For this review, take the finished solid that the model builds, in its own axes (mm). Face numbers are marked on the shaded views. A direction names the side the tool comes from. Round coordinates to 2 decimals unless told otherwise and drop trailing zeros. Write each loop counter-clockwise with the first axis right and the second up, starting at its lowest first coordinate (ties: lowest second). Pieces come first, ordered by that corner, then holes. Notation, with made-up numbers: (-25, 13.25) -> (0, 13.25) arc R12 cw to (0, 36.25) -> close; hole circle Ø10 at (8, 16.5). An arc over 180 degrees is marked (long way). Answer as CSV lines item,"result". Start each with the question number.
Item 1: Take a section at D-D on x = 31. Give the boundary of the cut face in (y, z), then the cut area to 3 significant figures.
Item 2: Take a section at B-B on z = -20. Count the separate pieces of the cut face and the enclosed holes in it, then the cut area to 3 significant figures.
Item 3: Wall thickness on probe 1 along X at (y, z) = (26.8, -20); probe 2 along Z at (x, y) = (21, 30.5); probe 3 along X at (y, z) = (27.5, -30): over which ranges is each line inside the solid? List them lowest first. Write a range as from..to.
Item 4: Mouldability with a two-part tool opening along Z and no side actions: class the marked faces 1, 2, 3 and 4 as +Z half, -Z half, draft (parallel to the pull), parting line (faces both ways), or undercut.
Item 5: For pin 1 Ø5.5 at (x, z) = (112.5, -22) entering from +Y; pin 2 Ø5 at (x, z) = (30.5, -30) entering from +Y; pin 3 Ø2.5 at (x, z) = (111.5, -19.5) entering from -Y; pin 4 Ø20 at (y, z) = (11.5, -22.5) entering from +X, all flat-tipped, find the tip position at first contact; note any pin that passes through.
Item 6: Machinability: for the marked faces 5 and 6, which of the approach directions +Z, -Z, +X, -X, +Y, -Y give a long, thin tool a straight path to every point of the face, cutting with its end or side? Answer none if there is none.
Item 7: Take a section at A-A on y = 2.5. Give the boundary of the cut face in (x, z), then the cut area to 3 significant figures.
Item 8: Take a section at C-C on z = -36.5. Give the boundary of the cut face in (x, y).
Autodesk Inventor part; units mm, degrees
ref_plane "YZ Plane" through (0, 0, 0) normal (1, 0, 0) x (0, 1, 0)
ref_plane "XZ Plane" through (0, 0, 0) normal (0, 1, 0) x (-1, 0, 0)
ref_plane "XY Plane" through (0, 0, 0) normal (0, 0, 1) x (1, 0, 0)
sketch "Sketch1" plane through (0, 0, 0) normal (0, 1, 0) x (-1, 0, 0)
  line L0 (0, 0) -> (-100, 0)
  line L1 (-100, 0) -> (-100, -40)
  line L2 (-100, -40) -> (0, -40)
  line L3 (0, -40) -> (0, 0)
  line L4 (2, -42) -> (-102, -42)
  line L5 (-102, -42) -> (-102, 2)
  line L6 (-102, 2) -> (2, 2)
  line L7 (2, 2) -> (2, -42)
  dimension "Length" = 100
  dimension "Width" = 40
  dimension "Thickness" = 2
extrude "Extrusion1" add sketch "Sketch1" along normal blind 40
sketch "Sketch2" plane through (0, 0, 0) normal (0, -1, 0) x (1, 0, 0)
  line L0 (102, -42) -> (102, 2)
  line L1 (102, 2) -> (-2, 2)
  line L2 (-2, -42) -> (102, -42)
  line L3 (-2, 2) -> (-2, -42)
  point P0 (0, 0)
extrude "Extrusion2" add sketch "Sketch2" along normal blind 2
sketch "Sketch3" plane through (-2, 40, -42) normal (-1, 0, 0) x (0, 0, 1)
  line L0 (0, 0) -> (44, 0)
  line L1 (19.5, -4) -> (24.5, -4)
  line L2 (24.5, -4) -> (24.5, -2)
  line L3 (24.5, -2) -> (19.5, -2)
  line L4 (19.5, -2) -> (19.5, -4)
  line L5 (19.5, -4) -> (24.5, -2) construction
  line L6 (24.5, -4) -> (19.5, -2) construction
  line L7 (22, -3) -> (22, 0) construction
  point P0 (42, -40)
  dimension "d7" = 5
  dimension "d8" = 2
  dimension "d9" = 2
extrude "Extrusion3" cut sketch "Sketch3" against normal up to next
sketch "Sketch4" plane through (102, 40, 2) normal (1, 0, 0) x (0, 0, -1)
  line L0 (14.5, -12) -> (29.5, -12)
  line L1 (29.5, -12) -> (29.5, -10)
  line L2 (29.5, -10) -> (14.5, -10)
  line L3 (14.5, -10) -> (14.5, -12)
  line L4 (14.5, -12) -> (29.5, -10) construction
  line L5 (29.5, -12) -> (14.5, -10) construction
  line L6 (0, 0) -> (44, 0)
  line L7 (22, -11) -> (22, 0) construction
  line L8 (44, 0) -> (0, 0)
  point P0 (2, -40)
  dimension "d12" = 10
  dimension "d13" = 15
  dimension "d14" = 2
extrude "Extrusion4" add sketch "Sketch4" along normal blind 10
sketch "Sketch5" plane through (102, 30, -12.5) normal (0, 1, 0) x (1, 0, 0)
  line L0 (0, 0) -> (0, 15)
  line L1 (0, 0) -> (10, 0)
  line L2 (10, 15) -> (10, 0)
  line L3 (0, 15) -> (10, 15)
  line L4 (10, 0) -> (10, 15)
  arc A0 (10, 0) -> (10, 15) centre (10, 7.5) ccw
  point P0 (-102, -12.5)
extrude "Extrusion5" add sketch "Sketch5" against normal blind 10
sketch "Sketch6" plane through (102, 30, -12.5) normal (0, 1, 0) x (1, 0, 0)
  arc A0 (10, 0) -> (10, 15) centre (10, 7.5) ccw
  point P0 (-102, -12.5)
hole "Hole1" at (112, 30, -20) direction (0, -1, 0) diameter 5.5 end through all
fillet "Fillet1" radius 2 11 edges at (119.5, 30, -20) (107, 30, -12.5) (107, 30, -27.5) (112, 30, -22.75) (119.5, 20, -20) (107, 20, -12.5) (107, 20, -27.5) (102, 25, -27.5) (102, 20, -20) (102, 25, -12.5) (102, 30, -20)
sketch "Sketch7" plane through (102, 20, -12.5) normal (0, -1, 0) x (1, 0, 0)
  circle A0 centre (10, -7.5) radius 2.75
  circle A1 centre (10, -7.5) radius 4 construction
  line L0 (14, -9.8094) -> (10, -12.1188)
  line L1 (10, -12.1188) -> (6, -9.8094)
  line L2 (6, -9.8094) -> (6, -5.1906)
  line L3 (6, -5.1906) -> (10, -2.8812)
  line L4 (10, -2.8812) -> (14, -5.1906)
  line L5 (14, -5.1906) -> (14, -9.8094)
  point P0 (-102, 12.5)
  point P1 (14, -7.5)
  dimension "d27" = 8
extrude "Extrusion6" cut sketch "Sketch7" against normal blind 3.5
equation "\"d5\" = Thickness"
equation "\"d10\" = Thickness"
equation "\"d14\" = Thickness"
properties part number "Casing_Part1"
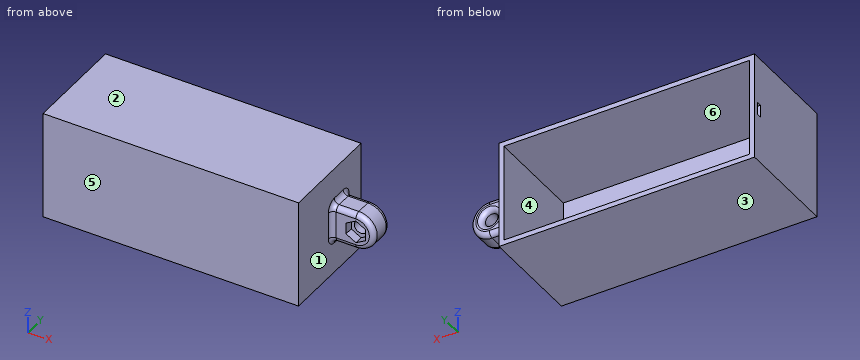
Output values:
1,outline,"(-2, -42) -> (40, -42) -> (40, -40) -> (0, -40) -> (0, 0) -> (40, 0) -> (40, 2) -> (-2, 2) -> close"
1,area,"248 mm^2"
2,separate pieces,"3"
2,enclosed holes,"0"
2,area,"474 mm^2"
3,probe 1,"x = -2..0, 100..109.25, 114.75..119.5"
3,probe 2,"z = -42..-40, 0..2"
3,probe 3,"x = -2..0, 100..102"
4,face 1,"draft"
4,face 2,"+Z half"
4,face 3,"-Z half"
4,face 4,"undercut"
5,pin 1,"stops at y = 30"
5,pin 2,"stops at y = 0"
5,pin 3,"passes through"
5,pin 4,"stops at x = 119.36"
6,face 5,"+Z, -Z, +X, -X, -Y"
6,face 6,"+Y"
7,outline,"(-2, -42) -> (102, -42) -> (102, 2) -> (-2, 2) -> close; hole (0, -40) -> (100, -40) -> (100, 0) -> (0, 0) -> close"
7,area,"576 mm^2"
8,outline,"(-2, -2) -> (102, -2) -> (102, 40) -> (100, 40) -> (100, 0) -> (0, 0) -> (0, 40) -> (-2, 40) -> close"
